Work out the finished part from the listing and answer in its coordinate system (mm). A direction names the side the tool comes from. Give positions to 0.01 mm unless a question says otherwise; leave off trailing zeros. Write each loop counter-clockwise with the first axis right and the second up, starting at its lowest first coordinate (ties: lowest second). Pieces come first, ordered by that corner, then holes. Notation, with made-up numbers: (-12.5, 41.5) - (32.5, 41.5) arc R17 cw to (32.5, 74.5) - close; hole circle Ø7 at (55, -31.75). An arc over 180 degrees is marked (long way). Write item = value, one per line.
from build123d import *

# Parameters (mm, degrees)
SKETCH1_W           = 35
SKETCH1_H           = 20
SKETCH1_R           = 1.625
SKETCH1_R_2         = 1.75
BOSS_EXTRUDE1_DEPTH = 6
CHAMFER1_SIZE       = 2.5
CUT_EXTRUDE1_DEPTH  = 2.5


with BuildPart() as part:
    # Sketch1 → Boss-Extrude1 (new body)
    with BuildSketch(Plane.XY):
        with Locations((17.5, 10)):
            Rectangle(SKETCH1_W, SKETCH1_H)
        with Locations((5, 10)):
            Circle(SKETCH1_R, mode=Mode.SUBTRACT)
        with Locations((30, 10)):
            Circle(SKETCH1_R_2, mode=Mode.SUBTRACT)
        with Locations((17.5, 10)):
            Circle(SKETCH1_R_2, mode=Mode.SUBTRACT)
    extrude(amount=BOSS_EXTRUDE1_DEPTH)

    # Chamfer1
    chamfer1_edges = [part.edges().sort_by_distance(p)[0] for p in [
        (3.375, 10, 6),
        (28.25, 10, 6),
    ]]
    chamfer(chamfer1_edges, length=CHAMFER1_SIZE)

    # Sketch2 → Cut-Extrude1 (cut)
    with BuildSketch(Plane(origin=(0, 0, 0), x_dir=(-1, 0, 0), z_dir=(0, 0, -1))):
        Polygon((-19.376388375, 13.25), (-21.25277675, 10), (-19.376388375, 6.75), (-15.623611625, 6.75), (-13.74722325, 10), (-15.623611625, 13.25), align=None)
    extrude(amount=-CUT_EXTRUDE1_DEPTH, mode=Mode.SUBTRACT)


solid = part.part
1. Find section D-D, the plane x = 17.5. Give the vertices of the cut face in (y, z), then the cut area to 3 significant figures.
Solution:
outline = (0, 0) - (6.75, 0) - (6.75, 2.5) - (8.25, 2.5) - (8.25, 6) - (0, 6) - close; (11.75, 2.5) - (13.25, 2.5) - (13.25, 0) - (20, 0) - (20, 6) - (11.75, 6) - close
area = 91.5 mm^2
2. A tool of negligible diameter and unlimited length cuts with its end or side. For faces 1 (the flat face through (0, 10, 3)), 2 (the flat face through (20.33, 8.4, 1.23)), from which of +Z, -Z, +X, -X, +Y, -Y can it reach the whole face along a straight path? Write none if from no direction.
Solution:
face_1 = +Z, -Z, -X, +Y, -Y
face_2 = -Z
3. Given pin 1 (4.5 mm diameter, centred on x = 30, y = 10, fed in from -Z); pin 2 (1 mm diameter, centred on x = 16, y = 9, fed in from -Z), each flat-ended and moving along its own axis, determine where each tip first touches the part or whether it passes through.
Solution:
pin_1 = 0
pin_2 = 2.5
4. Find section C-C, the plane x = 5. Give the vertices of the cut face in (y, z) (3 decimals).
Solution:
outline = (0, 0) - (8.375, 0) - (8.375, 3.5) - (5.875, 6) - (0, 6) - close; (11.625, 0) - (20, 0) - (20, 6) - (14.125, 6) - (11.625, 3.5) - close
5. Find section B-B, the plane z = 1.9. Give the vertices of the cut face in (x, y) (3 decimals), then the cut area to 3 significant figures.
Solution:
outline = (0, 0) - (35, 0) - (35, 20) - (0, 20) - close; hole circle Ø3.25 at (5, 10); hole (13.747, 10) - (15.624, 6.75) - (19.376, 6.75) - (21.253, 10) - (19.376, 13.25) - (15.624, 13.25) - close; hole circle Ø3.5 at (30, 10)
area = 645 mm^2
6. Straight lines are drawn through the part: line 1 (Y direction, x = 18, z = 2.2); line 2 (Y direction, x = 5, z = 1.7) (3 decimals); line 3 (X direction, y = 10, z = 5.05) (3 decimals). For each, find the intervals that lie inside material, in ascending order.
Solution:
line_1 = 0 to 6.75, 13.25 to 20
line_2 = 0 to 8.375, 11.625 to 20
line_3 = 0 to 1.825, 8.175 to 15.75, 19.25 to 26.7, 33.3 to 35
7. Find section A-A, the plane x = 30. Give the vertices of the cut face in (y, z), then the cut area to 4 significant figures.
Solution:
outline = (0, 0) - (8.25, 0) - (8.25, 3.5) - (5.75, 6) - (0, 6) - close; (11.75, 0) - (20, 0) - (20, 6) - (14.25, 6) - (11.75, 3.5) - close
area = 92.75 mm^2
8. For a pull along Y with two mould halves and no side action, classify faces 3 (the flat face through (35, 10, 3)), 4 (the flat face through (17, 0, 3)), 5 (the flat face through (18, 6.75, 1)) as pulls with the +Y half, pulls with the -Y half, needs draft (parallel to the pull), parting line crosses it, or undercut.
Solution:
face_3 = needs draft
face_4 = pulls with the -Y half
face_5 = undercut
